Source: three-view drawing plus pictorial views. Frame: mm from the lowest corner of the part. A direction names the side the tool comes from. Round coordinates to 2 decimals unless told otherwise and drop trailing zeros. Loops run counter-clockwise (first coordinate to the right, second up) from the corner with the lowest first, then second, coordinate; pieces in that order, holes last. Notation, with made-up numbers: (-20, 83) -> (-1, 83) arc R13 cw to (-1, 103) -> close; hole circle Ø11 at (84, 85). An arc over 180 degrees is marked (long way). Answer in a Markdown table with one row per item.
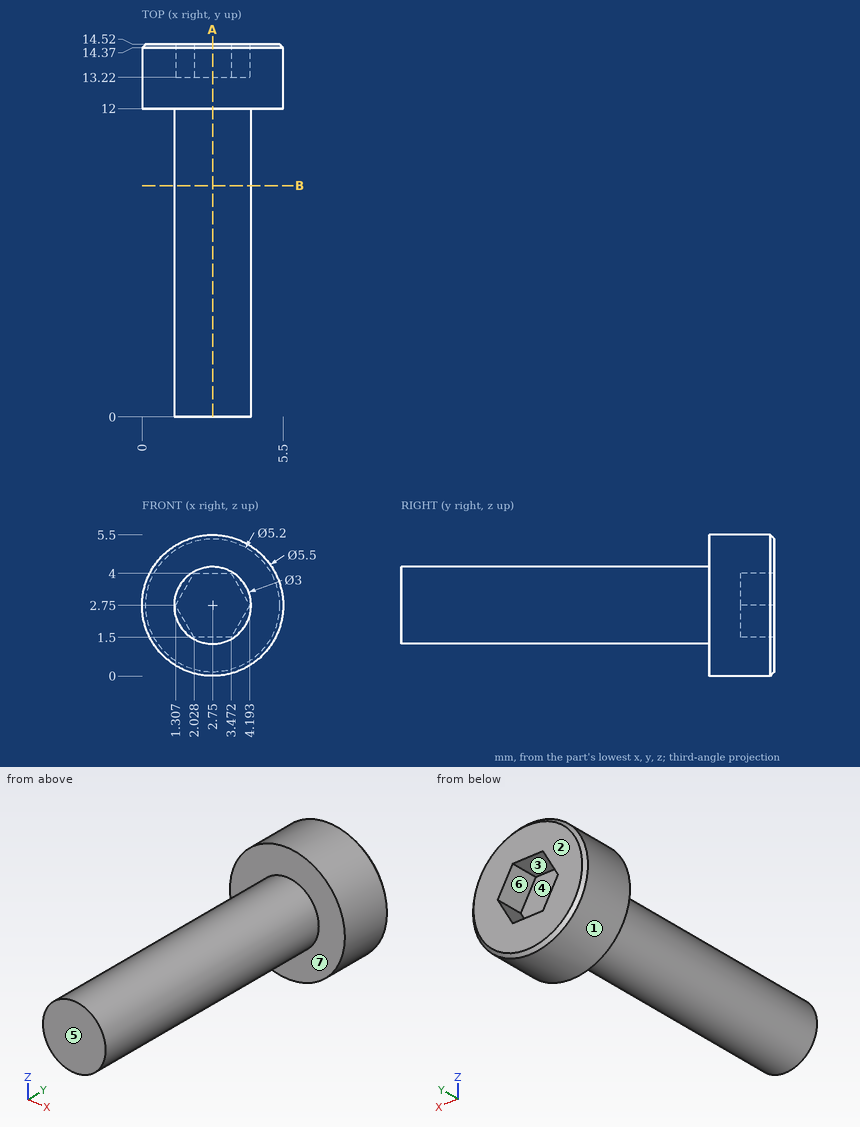
Item 1: Cut plane A-A (x = 2.75). Output: boundary loops of the cut face in (y, z).
Answer:
| item | result |
|---|---|
| outline | (0, 1.25) -> (12, 1.25) -> (12, 0) -> (14.37, 0) -> (14.52, 0.15) -> (14.52, 1.5) -> (13.22, 1.5) -> (13.22, 4) -> (14.52, 4) -> (14.52, 5.35) -> (14.37, 5.5) -> (12, 5.5) -> (12, 4.25) -> (0, 4.25) -> close |
Item 2: Pin query (flat end, axial travel): pin 1 Ø2 at (x, y) = (1, 12) entering from -Z (1 decimal); pin 2 Ø3 at (x, y) = (0.5, 4) entering from -Z; pin 3 Ø1.5 at (y, z) = (9, 2) entering from -X. Return the tip coordinate at first contact, or that it passes through.
Answer:
| item | result |
|---|---|
| pin 1 | stops at z = 0.1 |
| pin 2 | stops at z = 1.45 |
| pin 3 | stops at x = 1.25 |
Item 3: Line query: probe 1 along Y at (x, z) = (3.95, 4.8); probe 2 along Y at (x, z) = (2.1, 3.45); probe 3 along Z at (x, y) = (2.85, 1). Output: solid intervals per line, ascending. Write a range as [from, to].
Answer:
| item | result |
|---|---|
| probe 1 | y = [12, 14.52] |
| probe 2 | y = [0, 13.22] |
| probe 3 | z = [1.25, 4.25] |
Item 4: Cut plane B-B (y = 9). Output: boundary loops of the cut face in (x, z).
Answer:
| item | result |
|---|---|
| outline | circle Ø3 at (2.75, 2.75) |
Item 5: Reachability of the marked faces 5, 6 and 7 from +Z, -Z, +X, -X, +Y, -Y: full face, straight path, thin tool, end or side. Return the list, or none.
Answer:
| item | result |
|---|---|
| face 5 | +Z, -Z, +X, -X, -Y |
| face 6 | +Y |
| face 7 | -Y |
Item 6: Draft query along X for the marked faces 1, 2, 3 and 4. Return one class per face: pulls with the +X half, pulls with the -X half, needs draft (parallel to the pull), parting line crosses it, or undercut.
Answer:
| item | result |
|---|---|
| face 1 | parting line crosses it |
| face 2 | needs draft |
| face 3 | undercut |
| face 4 | undercut |
